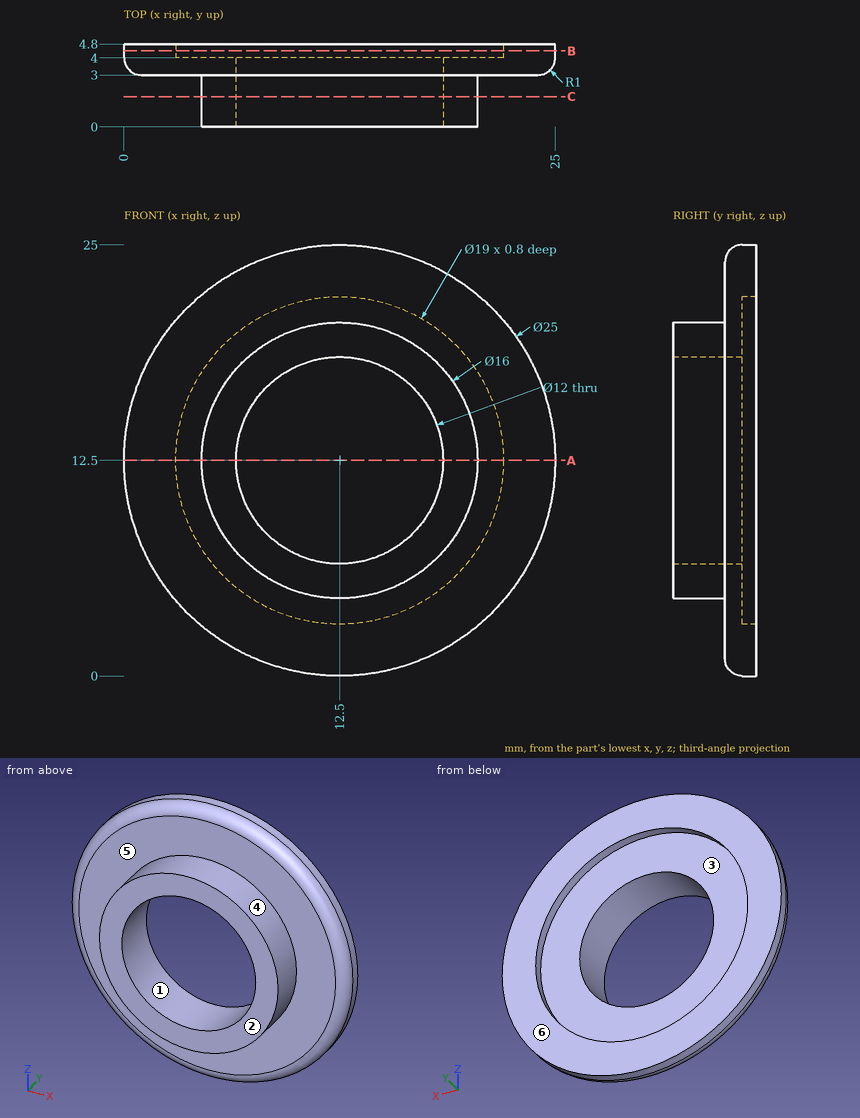
The drawing under review shows one solid part. Ordinate dimensions are in mm from its lowest x, y, z. A direction names the side the tool comes from. Give positions to 0.01 mm unless a question says otherwise; leave off trailing zeros. Write each loop counter-clockwise with the first axis right and the second up, starting at its lowest first coordinate (ties: lowest second). Pieces come first, ordered by that corner, then holes.
1. For P1, Ø1, axis at x = 14, z = 16.5, coming from the +Y side; P2, Ø1.5, axis at x = 4.5, z = 12.5, coming from the +Y side; P3, Ø2, axis at x = 21.5, z = 13.5, coming from the -Y side; P4, Ø1.5, axis at y = 2, z = 9, coming from the -X side, all flat-tipped, find the tip position at first contact; note any pin that passes through.
2. Add section C-C, the plane y = 1.75. Write out the cut boundary in (x, z), plus the area to 3 significant figures.
3. Wall thickness on L1, parallel to X at y = 2.1, z = 12.5; L2, parallel to X at y = 4.4, z = 12.5; L3, parallel to Y at x = 9, z = 20.5: over which ranges is each line inside the solid? List them lowest first.
4. Add section A-A, the plane z = 12.5. Write out the cut boundary in (x, y).
5. Draft analysis for pull direction Z (two halves, no side actions). For the marked faces 1, 2, 3 and 4, state which applies: +Z half, -Z half, draft (parallel to the pull), parting line (faces both ways), or undercut.
6. Add section B-B, the plane y = 4.4. Write out the cut boundary in (x, z), plus the area to 3 significant figures.
7. Tool access review of the marked faces 5 and 6: name each direction out of +Z, -Z, +X, -X, +Y, -Y from which nothing blocks a thin tool from reaching the whole face with its end or side.
Worked answers:
1. P1: passes through
1. P2: stops at y = 4
1. P3: stops at y = 3
1. P4: stops at x = 4.99
2. outline: circle Ø16 at (12.5, 12.5); hole circle Ø12 at (12.5, 12.5)
2. area: 88.0 mm2
3. L1: x = 4.5 to 6.5, 18.5 to 20.5
3. L2: x = 0 to 3, 22 to 25
3. L3: y = 3 to 4
4. outline: (0, 4) arc R1 ccw to (1, 3) - (4.5, 3) - (4.5, 0) - (6.5, 0) - (6.5, 4) - (3, 4) - (3, 4.8) - (0, 4.8) - close; (18.5, 0) - (20.5, 0) - (20.5, 3) - (24, 3) arc R1 ccw to (25, 4) - (25, 4.8) - (22, 4.8) - (22, 4) - (18.5, 4) - close
5. face 1: undercut
5. face 2: draft
5. face 3: undercut
5. face 4: parting line
6. outline: circle Ø25 at (12.5, 12.5); hole circle Ø19 at (12.5, 12.5)
6. area: 207 mm2
7. face 5: -Y
7. face 6: +Z, -Z, +X, -X, +Y
